Geometry check sheet. Reference: the model listing, model coordinates, mm. A direction names the side the tool comes from. Give positions to 0.01 mm unless a question says otherwise; leave off trailing zeros. Write each loop counter-clockwise with the first axis right and the second up, starting at its lowest first coordinate (ties: lowest second). Pieces come first, ordered by that corner, then holes. Notation, with made-up numbers: (77.25, -28) - (100.25, -28) arc R4 ccw to (100.25, -24) - close; hole circle Ø6 at (45.5, -32). An arc over 180 degrees is marked (long way). Use a Markdown table: item, result.
Autodesk Inventor part; units mm, degrees
ref_plane "YZ Plane" through (0, 0, 0) normal (1, 0, 0) x (0, 1, 0)
ref_plane "XZ Plane" through (0, 0, 0) normal (0, 1, 0) x (-1, 0, 0)
ref_plane "XY Plane" through (0, 0, 0) normal (0, 0, 1) x (1, 0, 0)
sketch "Sketch1" plane through (0, 0, 0) normal (0, 1, 0) x (-1, 0, 0)
  line L0 (-19.05, 19.05) -> (19.05, 19.05)
  line L1 (19.05, 19.05) -> (19.05, -19.05)
  line L2 (19.05, -19.05) -> (-19.05, -19.05)
  line L3 (-19.05, -19.05) -> (-19.05, 19.05)
  line L4 (-19.05, 19.05) -> (19.05, -19.05) construction
  line L5 (19.05, 19.05) -> (-19.05, -19.05) construction
  line L6 (17.4625, -17.4625) -> (17.4625, 17.4625)
  line L7 (17.4625, 17.4625) -> (-17.4625, 17.4625)
  line L8 (-17.4625, 17.4625) -> (-17.4625, -17.4625)
  line L9 (-17.4625, -17.4625) -> (17.4625, -17.4625)
  point P0 (0, 0)
  dimension "d0" = 38.1
  dimension "d1" = 1.5875
extrude "Extrusion1" add sketch "Sketch1" along normal mid plane 812.8
sketch "Sketch2" plane through (19.05, -406.4, -19.05) normal (1, 0, 0) x (0, 0, -1)
  circle A0 centre (-25.4, 806.45) radius 2.4892
  circle A1 centre (-25.4, 793.75) radius 2.4892
  circle A2 centre (-12.7, 793.75) radius 2.4892
  circle A3 centre (-12.7, 806.45) radius 2.4892
  line L0 (-38.1, 812.8) -> (0, 812.8)
  circle A4 centre (-31.75, 12.7) radius 2.4892
  circle A5 centre (-6.35, 12.7) radius 2.4892
  circle A6 centre (-6.35, 79.375) radius 2.4892
  circle A7 centre (-31.75, 79.375) radius 2.4892
  line L1 (0, 0) -> (-38.1, 0)
  line L2 (-38.1, 0) -> (-38.1, 812.8)
  point P0 (-19.05, 800.1)
  point P1 (-19.05, 812.8)
  dimension "d4" = 4.9784
  dimension "d7" = 360
  dimension "d9" = 12.7
  dimension "d10" = 6.35
  dimension "d11" = 4.9784
  dimension "d12" = 66.675
  dimension "d13" = 12.7
  dimension "d14" = 25.4
  dimension "d15" = 6.35
extrude "Extrusion2" cut sketch "Sketch2" against normal through all
sketch "Sketch3" plane through (-19.05, 406.4, 19.05) normal (0, 0, 1) x (1, 0, 0)
  line L0 (0, 0) -> (38.1, 0)
  line L1 (7.9375, 0) -> (7.9375, -6.35)
  line L2 (7.9375, -6.35) -> (30.1625, -6.35)
  line L3 (30.1625, -6.35) -> (30.1625, 0)
  point P0 (19.05, -6.35)
  point P1 (19.05, 0)
  dimension "d18" = 22.225
  dimension "d19" = 6.35
extrude "Extrusion3" cut sketch "Sketch3" against normal through all
fillet "Fillet1" radius 2.54 8 edges at (-11.1125, 406.4, 18.2562) (-11.1125, 400.05, 18.2562) (11.1125, 400.05, 18.2562) (11.1125, 406.4, 18.2562) (-11.1125, 406.4, -18.2562) (-11.1125, 400.05, -18.2562) (11.1125, 406.4, -18.2562) (11.1125, 400.05, -18.2562)
properties part number "GreyT 2x1 Template" material "Aluminum 6061"
1) Section check A-A on x = -2. Record the boundary of the cut face in (y, z), then the cut area to 3 significant figures.
Working result:
| item | result |
|---|---|
| outline | (-406.4, -19.05) - (400.05, -19.05) - (400.05, -17.46) - (-406.4, -17.46) - close; (-406.4, 17.46) - (400.05, 17.46) - (400.05, 19.05) - (-406.4, 19.05) - close |
| area | 2,560 mm² |
2) Depth check by flat-ended pin: P1, Ø4.5, axis at y = 400.05, z = 6.35, coming from the +X side; P2, Ø1.7, axis at x = 2, z = -18.5, coming from the +Y side. Enter the tip coordinate at first touch or a pass-through.
Working result:
| item | result |
|---|---|
| P1 | passes through |
| P2 | stops at y = 400.05 |
3) Set-up check for faces 1 (the flat face through (0, -6, 17.462)), 2 (the flat face through (-19.05, -6, 0)): record each of +Z, -Z, +X, -X, +Y, -Y from which the full face is reachable in a straight line by a thin tool's end or side.
Working result:
| item | result |
|---|---|
| face 1 | +Y, -Y |
| face 2 | +Z, -Z, -X, +Y, -Y |
4) Section check B-B on y = 170. Record the boundary of the cut face in (x, z).
Working result:
| item | result |
|---|---|
| outline | (-19.05, -19.05) - (19.05, -19.05) - (19.05, 19.05) - (-19.05, 19.05) - close; hole (-17.46, -17.46) - (17.46, -17.46) - (17.46, 17.46) - (-17.46, 17.46) - close |
5) Material ranges on L1, parallel to Y at x = 18.2, z = 6.35; L2, parallel to Z at x = -17.85, y = -393.7; L3, parallel to Z at x = 18, y = 387, recorded low to high. Write a range as from..to.
Working result:
| item | result |
|---|---|
| L1 | y = -406.4..384.86, 389.84..397.56, 402.54..406.4 |
| L2 | z = -19.05..-15.19, -10.21..10.21, 15.19..19.05 |
| L3 | z = -19.05..-8.81, -3.89..3.89, 8.81..19.05 |
6) Mould release check, pull along Z, two halves, no side actions. Record for faces 3 (the flat face through (2, -406.4, -18)), 4 (the flat face through (0, -6, -19.05)), 5 (the flat face through (0, -6, 19.05)), 6 (the flat face through (-17.462, -6, 0)): pulls with the +Z half, pulls with the -Z half, needs draft (parallel to the pull), parting line crosses it, or undercut.
Working result:
| item | result |
|---|---|
| face 3 | needs draft |
| face 4 | pulls with the -Z half |
| face 5 | pulls with the +Z half |
| face 6 | undercut |
